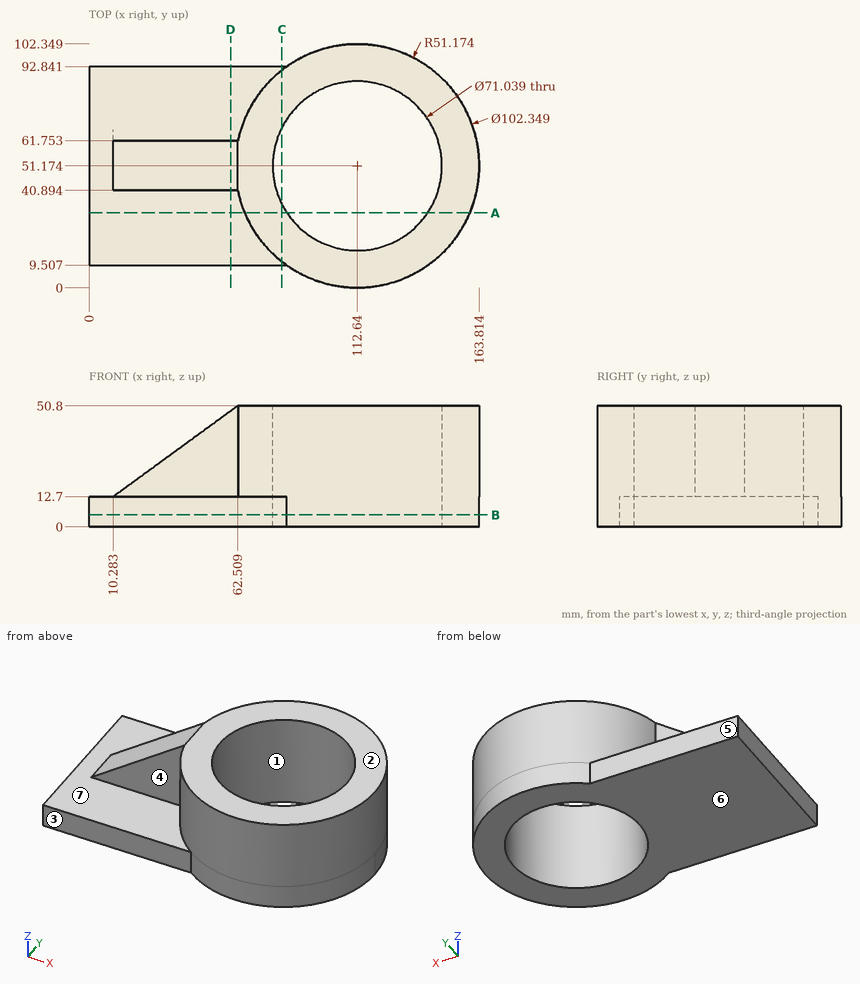
Verification items for this drawing (mm, ordinates from the low corner). A direction names the side the tool comes from. Coordinates: 2 decimals unless noted, no trailing zeros. Order: outer loops, then holes, each group sorted by start corner. A loop starts at its lowest first (then second) coordinate and runs counter-clockwise, first axis right, second up. Notation, with made-up numbers: M 0,-9.5 L 34,-9.5 A20 cw 34,-5.5 Z; hole C -13,24.5 d5. An arc over 180 degrees is marked long. Answer as a JSON object with one key per item and string values.
Q1. Cross-section at A-A on y = 31.5. Record the cut outline in (x, z), and give its area (3 significant figures).
Results are:
{"outline": "M 0,0 L 83.07,0 L 83.07,50.8 L 65.4,50.8 L 65.4,12.7 L 0,12.7 Z; M 142.21,0 L 159.88,0 L 159.88,50.8 L 142.21,50.8 Z", "area": "2,630 mm²"}
Q2. Depth check by flat-ended pin: pin 1 Ø6 at (y, z) = (88.5, 38.5) entering from -X (1 decimal); pin 2 Ø6.5 at (x, z) = (53.5, 6) entering from +Y; pin 3 Ø12 at (y, z) = (79.5, 28.5) entering from +X. Enter the tip coordinate at first touch or a pass-through.
Results are:
{"pin 1": "stops at x = 74.7", "pin 2": "stops at y = 92.84", "pin 3": "stops at x = 158.69"}
Q3. Cross-section at D-D on x = 59.5. Record the cut outline in (y, z) (1 decimal), and give its area (3 significant figures).
Results are:
{"outline": "M 9.5,0 L 92.8,0 L 92.8,12.7 L 61.8,12.7 L 61.8,48.6 L 40.9,48.6 L 40.9,12.7 L 9.5,12.7 Z", "area": "1,810 mm²"}
Q4. Cross-section at B-B on z = 5. Record the cut outline in (x, y) (1 decimal).
Results are:
{"outline": "M 0,9.5 L 82.9,9.5 A51.2 ccw long 82.9,92.8 L 0,92.8 Z; hole C 112.6,51.2 d71"}
Q5. Scan lines: line 1 (Y direction, x = 87, z = 34) (1 decimal); line 2 (X direction, y = 70, z = 14) (1 decimal); line 3 (Y direction, x = 34.5, z = 29). Record each from-to range of solid material in increasing order.
Results are:
{"line 1": "y = 6.9 to 26.6, 75.8 to 95.5", "line 2": "x = 65.1 to 82.5, 142.8 to 160.2", "line 3": "y = 40.89 to 61.75"}
Q6. Cross-section at C-C on x = 81. Record the cut outline in (y, z) (1 decimal).
Results are:
{"outline": "M 9.5,0 L 35,0 L 35,50.8 L 11,50.8 L 11,12.7 L 9.5,12.7 Z; M 67.3,0 L 92.8,0 L 92.8,12.7 L 91.4,12.7 L 91.4,50.8 L 67.3,50.8 Z"}
Q7. Release check for a two-part mould opening along Y. For the marked faces 1, 2 and 3 record: released by +Y, released by -Y, zero draft, split by the parting line, or undercut.
Results are:
{"face 1": "undercut", "face 2": "zero draft", "face 3": "released by -Y"}
Q8. Tool access check on the marked faces 4, 5, 6 and 7. Record the directions out of +Z, -Z, +X, -X, +Y, -Y that give a thin tool (end or side, any length) a straight path to the whole face; none if there is none.
Results are:
{"face 4": "+Z, -X, -Y", "face 5": "+Z, -Z, -X, +Y", "face 6": "-Z, +X, -X, +Y, -Y", "face 7": "+Z, -X"}
